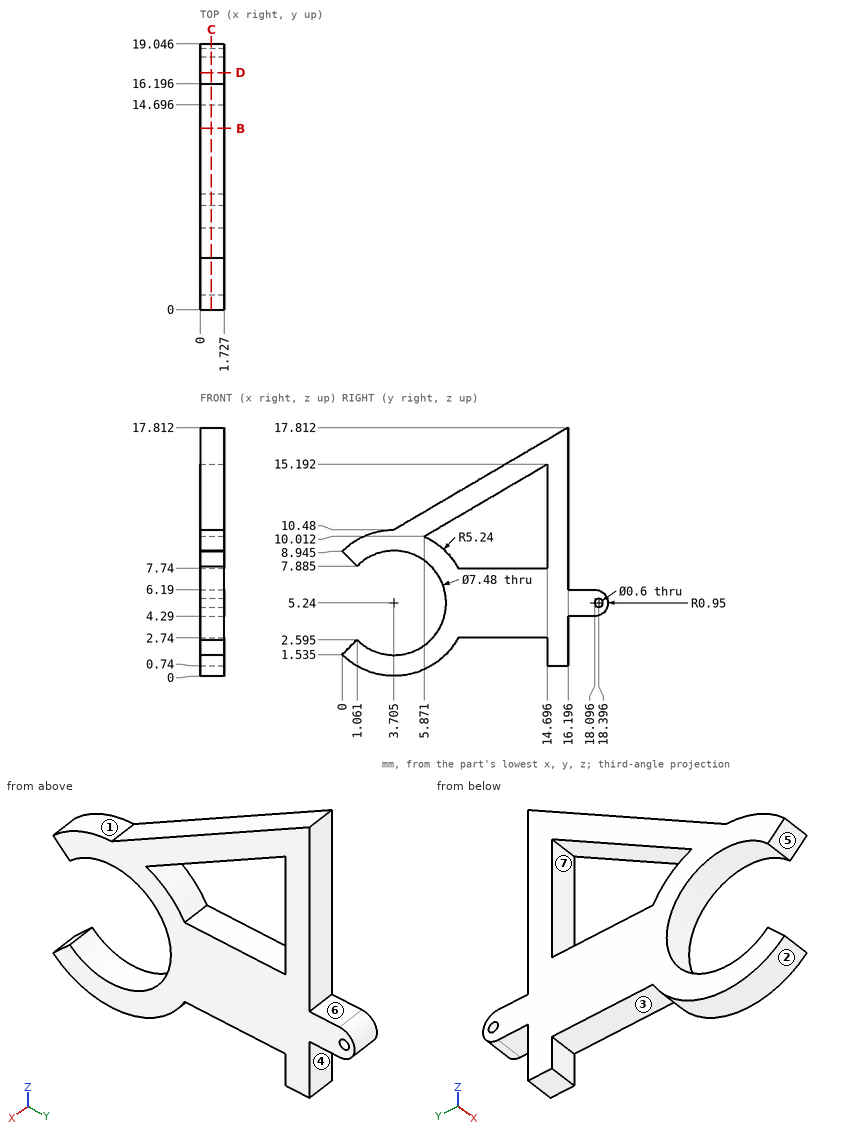
The figure shows three views and two pictorial views of one solid part (mm, origin at its lowest corner). Answer the questions. A direction names the side the tool comes from. Round coordinates to 2 decimals unless told otherwise and drop trailing zeros. Write each loop counter-clockwise with the first axis right and the second up, starting at its lowest first coordinate (ties: lowest second). Pieces come first, ordered by that corner, then holes. Notation, with made-up numbers: (50, 89) -> (68, 89) arc R14 ccw to (68, 98) -> close; hole circle Ø5 at (13, 11). An arc over 180 degrees is marked (long way). Answer as a JSON object with one key per item and string values. Group by question number.
Q1. Section C-C (x = 0.8) is taken. Count the separate pieces of the cut face and the enclosed holes in it, plus the area to 3 significant figures.
Q2. Section B-B (y = 13) is taken. Write down the section's boundary in (x, z) (1 decimal).
Q3. Which of the six approach directions +Z, -Z, +X, -X, +Y, -Y give full straight-line access (tool end or side, diameter ignored) to the marked faces 5, 6 and 7?
Q4. Section D-D (y = 17) is taken. Write down the section's boundary in (x, z).
Q5. Each of these flat-tipped pins is pushed along its axis until it touches: pin 1 Ø0.9 at (x, y) = (1, 17) entering from -Z; pin 2 Ø0.5 at (x, y) = (0.5, 11.5) entering from -Z; pin 3 Ø0.5 at (x, z) = (1, 13) entering from +Y. Where does it stop, or does it pass through?
Q6. Determine the mould class of the marked faces 1, 2, 3 and 4 for opening direction Y: pulls with the +Y half, pulls with the -Y half, needs draft (parallel to the pull), parting line crosses it, or undercut.
Q7. Straight lines are drawn through the part: line 1 along Y through (x, z) = (1, 2) (1 decimal); line 2 along Z through (x, y) = (0.25, 17); line 3 along Y through (x, z) = (1.2, 12.25) (1 decimal). For each, find the intervals that lie inside material, in ascending order.
Check values:
{
 "1": {"separate pieces": "1", "enclosed holes": "2", "area": "108 mm^2"},
 "2": {"outline": "(0, 2.7) -> (1.7, 2.7) -> (1.7, 7.7) -> (0, 7.7) -> close; (0, 14.2) -> (1.7, 14.2) -> (1.7, 15.9) -> (0, 15.9) -> close"},
 "3": {"face 5": "+X, -X, -Y", "face 6": "+Z, +X, -X, +Y", "face 7": "+X, -X"},
 "4": {"outline": "(0, 4.29) -> (1.73, 4.29) -> (1.73, 6.19) -> (0, 6.19) -> close"},
 "5": {"pin 1": "z = 4.29", "pin 2": "z = 2.74", "pin 3": "y = 16.2"},
 "6": {"face 1": "pulls with the -Y half", "face 2": "undercut", "face 3": "undercut", "face 4": "pulls with the +Y half"},
 "7": {"line 1": "0.5 to 1.8, 5.6 to 7.8, 14.7 to 16.2", "line 2": "4.29 to 6.19", "line 3": "6.7 to 9.7, 14.7 to 16.2"}
}
